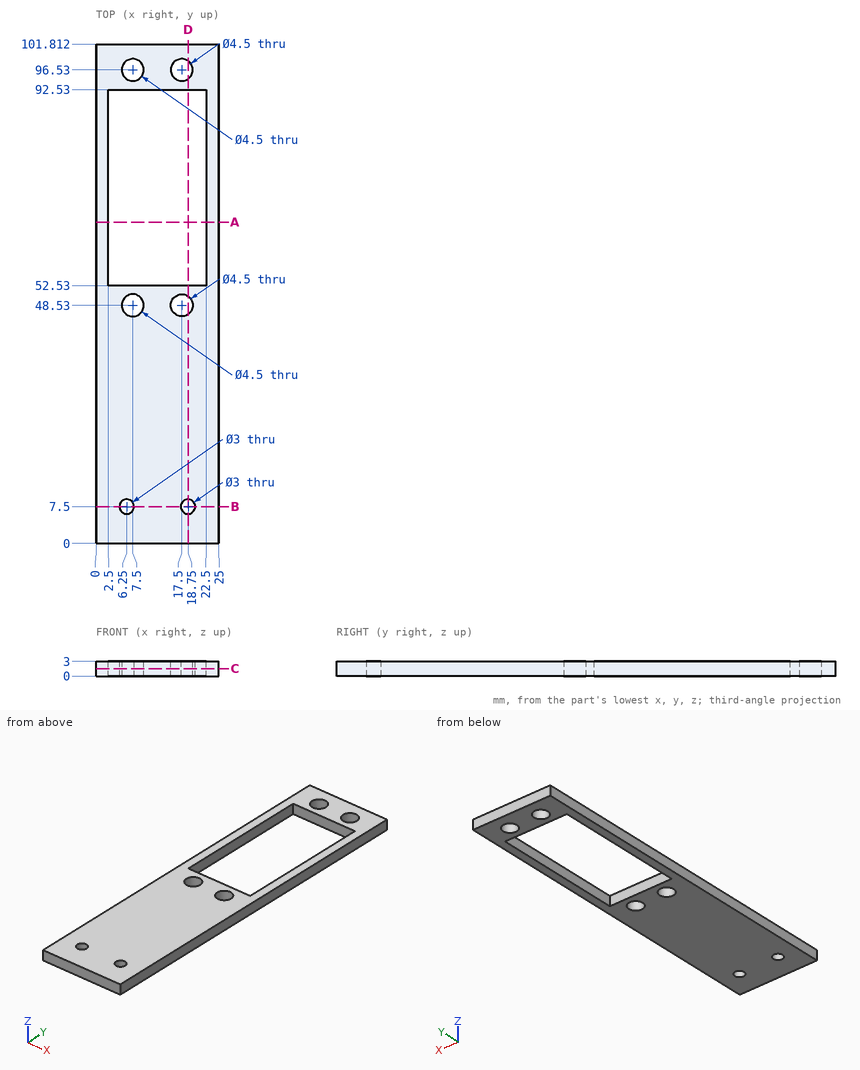
Could you check a few things on this drawing? It's one solid part, dimensions in mm from its lowest x, y, z. Coordinates: 2 decimals unless noted, no trailing zeros. Order: outer loops, then holes, each group sorted by start corner. A loop starts at its lowest first (then second) coordinate and runs counter-clockwise, first axis right, second up. Notation, with made-up numbers: M -13,-35.5 L 22,-35.5 A18 cw 22,-0.5 Z; hole C -3,18 d4. An arc over 180 degrees is marked long. Answer as CSV lines item,"result".
(1) Suppose I cut it at C-C on z = 1.5. Please give me the cut outline in (x, y), plus the area to 3 significant figures.
Geometry check:
outline,"M 0,0 L 25,0 L 25,101.81 L 0,101.81 Z; hole M 2.5,52.53 L 22.5,52.53 L 22.5,92.53 L 2.5,92.53 Z; hole C 6.25,7.5 d3; hole C 7.5,48.53 d4.5; hole C 7.5,96.53 d4.5; hole C 17.5,48.53 d4.5; hole C 17.5,96.53 d4.5; hole C 18.75,7.5 d3"
area,"1,670 mm^2"
(2) Please list where these lines run through material, in increasing order: L1, parallel to X at y = 59.5, z = 2.15; L2, parallel to Y at x = 12.5, z = 0.5; L3, parallel to Y at x = 7.5, z = 1.5.
Geometry check:
L1,"0 to 2.5, 22.5 to 25"
L2,"0 to 52.53, 92.53 to 101.81"
L3,"0 to 6.67, 8.33 to 46.28, 50.78 to 52.53, 92.53 to 94.28, 98.78 to 101.81"
(3) Suppose I cut it at B-B on y = 7.5. Please give me the cut outline in (x, z).
Geometry check:
outline,"M 0,0 L 4.75,0 L 4.75,3 L 0,3 Z; M 7.75,0 L 17.25,0 L 17.25,3 L 7.75,3 Z; M 20.25,0 L 25,0 L 25,3 L 20.25,3 Z"
(4) Suppose I cut it at A-A on y = 65.5. Please give me the cut outline in (x, z).
Geometry check:
outline,"M 0,0 L 2.5,0 L 2.5,3 L 0,3 Z; M 22.5,0 L 25,0 L 25,3 L 22.5,3 Z"
(5) I'm going to push flat-ended pins straight in: pin 1 (3.5 mm diameter, centred on x = 6.25, y = 7.5, fed in from +Z); pin 2 (2.5 mm diameter, centred on x = 18.75, y = 7.5, fed in from -Z). Where does each tip first touch, or does it pass through?
Geometry check:
pin 1,"z = 3"
pin 2,"through"
(6) Suppose I cut it at D-D on x = 18.75. Please give me the cut outline in (y, z), plus the area to 3 significant figures.
Geometry check:
outline,"M 0,0 L 6,0 L 6,3 L 0,3 Z; M 9,0 L 46.66,0 L 46.66,3 L 9,3 Z; M 50.4,0 L 52.53,0 L 52.53,3 L 50.4,3 Z; M 92.53,0 L 94.66,0 L 94.66,3 L 92.53,3 Z; M 98.4,0 L 101.81,0 L 101.81,3 L 98.4,3 Z"
area,"154 mm^2"
